from build123d import *

# Parameters (mm, degrees)
CLINCHINGRINGSEGMENT_DEPTH = 0.38608
CLINCHINGRING_COUNT        = 24
CLINCHINGRING_ANGLE        = 345
SQRCUT_DEPTH               = 0.9652


with BuildPart() as part:
    # BodySke → Body (revolve)
    with BuildSketch(Plane.XY, mode=Mode.PRIVATE) as body_sk:
        with BuildLine():
            Line((6.304896608, 0), (7.62, 0))
            Line((7.62, 0), (7.62, 2.667))
            Line((7.62, 2.667), (6.477, 2.667))
            Line((6.477, 2.667), (6.477, 3.683))
            ThreePointArc((6.477, 3.683), (5.993433296, 4.850433296), (4.826, 5.334))
            Line((4.826, 5.334), (4.191, 5.334))
            Line((4.191, 5.334), (4.191, 4.7752))
            Line((4.191, 4.7752), (3.81, 4.7752))
            Line((3.81, 4.7752), (3.538890129, 7.874))
            Line((3.538890129, 7.874), (2.5527, 7.874))
            Line((2.5527, 7.874), (2.5527, -0.9652))
            Line((2.5527, -0.9652), (6.5278, -0.9652))
            Line((6.5278, -0.9652), (6.5278, -0.77216))
            Line((6.5278, -0.77216), (6.304896608, -0.38608))
            Line((6.304896608, -0.38608), (6.304896608, 0))
        make_face()
    revolve(body_sk.sketch.rotate(Axis((0, 0, 0), (0, 1, 0)), 90), axis=Axis((0, 0, 0), (0, 1, 0)))

    # EndChamferSke → EndChamfer (revolve, cut)
    with BuildSketch(Plane.XY, mode=Mode.PRIVATE) as endchamfer_sk:
        Polygon((3.175, -1.2192), (3.175, -0.96266), (2.5527, -0.527082692), (2.5527, -1.2192), align=None)
        Polygon((3.175, 7.874), (2.5527, 7.438422692), (2.5527, 7.874), align=None)
    revolve(endchamfer_sk.sketch.rotate(Axis((0, -2.54, 0), (0, 1, 0)), 90), axis=Axis((0, -2.54, 0), (0, 1, 0)), mode=Mode.SUBTRACT)

    # CliRinSegSke → ClinchingRingSegment (add)
    with BuildSketch(Plane.XZ):
        Polygon((0.944879105, 7.177069351), (0, 6.858), (-0.944879105, 7.177069351), (-0.916532732, 6.961757271), (0, 6.65226), (0.916532732, 6.961757271), align=None)
    clinchingringsegment = extrude(amount=CLINCHINGRINGSEGMENT_DEPTH)

    # ClinchingRing: ClinchingRingSegment ×24 about axis
    clinchingring_axis = Axis((0, 0, 0), (0, 1, 0))
    for i in range(1, CLINCHINGRING_COUNT):
        add(clinchingringsegment.rotate(clinchingring_axis, i * CLINCHINGRING_ANGLE / (CLINCHINGRING_COUNT - 1)))

    # SqrCutSke → SqrCut (cut)
    with BuildSketch(Plane.XZ.offset(0.9652)):
        with BuildLine():
            Line((-3.556, -4.191), (3.556, -4.191))
            ThreePointArc((3.556, -4.191), (4.005012806, -4.005012806), (4.191, -3.556))
            Line((4.191, -3.556), (4.191, 3.556))
            ThreePointArc((4.191, 3.556), (4.005012806, 4.005012806), (3.556, 4.191))
            Line((3.556, 4.191), (-3.556, 4.191))
            ThreePointArc((-3.556, 4.191), (-4.005012806, 4.005012806), (-4.191, 3.556))
            Line((-4.191, 3.556), (-4.191, -3.556))
            ThreePointArc((-4.191, -3.556), (-4.005012806, -4.005012806), (-3.556, -4.191))
        make_face()
        with BuildLine():
            Line((3.81, -3.556), (3.81, 3.556))
            ThreePointArc((3.81, 3.556), (3.735605122, 3.735605122), (3.556, 3.81))
            Line((3.556, 3.81), (-3.556, 3.81))
            ThreePointArc((-3.556, 3.81), (-3.735605122, 3.735605122), (-3.81, 3.556))
            Line((-3.81, 3.556), (-3.81, -3.556))
            ThreePointArc((-3.81, -3.556), (-3.735605122, -3.735605122), (-3.556, -3.81))
            Line((-3.556, -3.81), (3.556, -3.81))
            ThreePointArc((3.556, -3.81), (3.735605122, -3.735605122), (3.81, -3.556))
        make_face(mode=Mode.SUBTRACT)
    extrude(amount=-SQRCUT_DEPTH, mode=Mode.SUBTRACT)


solid = part.part
Here's how the part is built. I have some questions about the finished solid (model axes, mm). A direction names the side the tool comes from. Round coordinates to 2 decimals unless told otherwise and drop trailing zeros. Order: outer loops, then holes, each group sorted by start corner. A loop starts at its lowest first (then second) coordinate and runs counter-clockwise, first axis right, second up. Notation, with made-up numbers: M -1,50.5 L 25,50.5 A13 cw 25,71.5 Z; hole C -3,32 d5. An arc over 180 degrees is marked long. Return JSON: item names as keys, results as strings. Group by question number.
1. If we section it at A-A on y = 1.25: List the corners of the cut face in (x, z) for me, then the cut area to 3 significant figures.
2. Please list where these lines run through material, in increasing order: probe 1 along X at (y, z) = (1.5, 0); probe 2 along Y at (x, z) = (4.25, -1); probe 3 along Y at (x, z) = (-4, -5.5).
3. On a 3-axis mill with a long thin cutter (end or side, diameter ignored), from which of +Z, -Z, +X, -X, +Y, -Y can I reach the whole of each face in a straight line? I mean faces 3 (the face through (-4.191, -0.5, 0)), 4 (the face through (-1.894, -0.19, -6.014)), 5 (the face through (-2, 5.334, 4)), 6 (the face through (-0.1, -0.965, -3.4)). Say none if no direction works.
4. I'm going to push flat-ended pins straight in: pin 1 Ø2 at (y, z) = (5.5, 2) entering from -X; pin 2 Ø2 at (x, y) = (-2.5, 2) entering from -Z; pin 3 Ø0.8 at (y, z) = (-0.5, 1.5) entering from -X. Where does each tip first touch, or does it pass through?
5. If we mould it in two halves opening along Z, with no side actions, what happens to faces 1 (the face through (6, 2.667, 3)), 2 (the face through (4.09, 5.05, 0.91))? For each: pulls with the +Z half, pulls with the -Z half, needs draft (parallel to the pull), parting line crosses it, or undercut.
Reply:
{
 "1": {"outline": "C 0,0 d15.24; hole C 0,0 d5.11", "area": "162 mm^2"},
 "2": {"probe 1": "-7.62 to -2.55, 2.55 to 7.62", "probe 2": "-0.97 to 5.33", "probe 3": "0 to 2.67"},
 "3": {"face 3": "-Y", "face 4": "none", "face 5": "+Y", "face 6": "+Z, -Z, +X, -X, -Y"},
 "4": {"pin 1": "x = -6", "pin 2": "z = -7.47", "pin 3": "x = -7.06"},
 "5": {"face 1": "needs draft", "face 2": "undercut"}
}
